Verification items for the finished model (mm, model axes). Face numbers are marked on the shaded views. A direction names the side the tool comes from. Coordinates: 2 decimals unless noted, no trailing zeros. Loops run counter-clockwise (first coordinate to the right, second up) from the corner with the lowest first, then second, coordinate; pieces in that order, holes last.
Q1. Access from +Z, -Z, +X, -X, +Y, -Y to the whole of each face (thin tool, end or side, straight path). Record for the marked faces 4 and 5.
Q2. Mould release check, pull along Z, two halves, no side actions. Record for the marked faces 1, 2 and 3: +Z half, -Z half, draft (parallel to the pull), parting line (faces both ways), or undercut.
Q3. Material ranges on probe 1 along Z at (x, y) = (-12.5, -12.25); probe 2 along X at (y, z) = (-2.5, -1); probe 3 along Z at (x, y) = (1.5, -8), recorded low to high.
Q4. Sectioned sample at A-A (x = 1). Enter the section's corners in (y, z).
Q5. Sectioned sample at B-B (z = 51). Enter the section's corners in (x, y), then the cut area to 3 significant figures.
Q6. Sectioned sample at D-D (y = -7). Count the separate pieces of the cut face and the enclosed holes in it, then the cut area to 3 significant figures.
Q7. Sectioned sample at C-C (z = 16). Enter the section's corners in (x, y).
Q8. Go/stop test with flat-tipped pins: P1, Ø0.9, axis at x = -12, z = 24.5, coming from the +Y side; P2, Ø0.5, axis at y = -7, z = 36.5, coming from the +X side; P3, Ø0.5, axis at x = -28.5, z = 46, coming from the +Y side. Record where each tip stops, or that it passes through.
```python
from build123d import *

# Parameters (mm, degrees)
BOSS_EXTRUDE1_DEPTH            = 77
SKETCH3_W                      = 37.54
SKETCH3_H                      = 17.27
BOSS_EXTRUDE2_DEPTH            = 1.77
SKETCH4_W                      = 37.54
SKETCH4_H                      = 17.27
BOSS_EXTRUDE3_DEPTH            = 1.77
SKETCH5_W                      = 4
SKETCH5_H                      = 16
CUT_EXTRUDE2_DEPTH             = 1.77
SKETCH6_W                      = 9.78
SKETCH6_H                      = 11.05
SKETCH6_W_2                    = 7.24
SKETCH6_H_2                    = 7.24
BUTTON_WALLS_DEPTH             = 7.24
SKETCH7_W                      = 9.78
SKETCH7_H                      = 11.05
BUTTON_BOTTOM_DEPTH            = 1.27
SKETCH8_W                      = 7.24
SKETCH8_H                      = 1.77
BUTTON_CUTOUT_MIDDLE_DEPTH     = 7.24
SKETCH9_W                      = 4.45
SKETCH9_H                      = 1.27
SKETCH9_W_2                    = 3.37
SKETCH9_H_2                    = 4.39
BUTTON_CUTOUT_FRONT_BACK_DEPTH = 7.24
SKETCH10_W                     = 3.37
SKETCH10_H                     = 4.39
BUTTON_CUTOUT_BOTTOM_DEPTH     = 1.27
BUTTON_CHAMFER1_SIZE           = 5
SKETCH12_W                     = 35
SKETCH12_H                     = 1.77
SKETCH12_W_2                   = 1.77
SKETCH12_H_2                   = 10
SKETCH12_W_3                   = 7.5
SKETCH12_R                     = 0.9652
SKETCH12_H_3                   = 7
SUPPORT_PCB_BATTERY_DEPTH      = 7
SKETCH13_R                     = 1.25
SKETCH13_W                     = 12
SKETCH13_H                     = 9
CUTOUT_USB_3_LEDS_DEPTH        = 1.77
SKETCH16_W                     = 1.77
SKETCH16_H                     = 1.77
TAB_PCB_RETAINER_LEN_DEPTH     = 3
SKETCH17_W                     = 4
SKETCH17_H                     = 1.77
CUTOUT_BACK_MOT_WIRES_DEPTH    = 9
SKETCH18_R                     = 1.25
CUTOUT_CHG_DONE_LED_DEPTH      = 10
SKETCH19_W                     = 4.2
SKETCH19_H                     = 1.77
TAB_PCB_RETAINERS_WIDTH_DEPTH  = 10
CUTOUT_RETAINER_TAB_1_DEPTH    = 1.77
CUTOUT_RETAINER_TAB_2_DEPTH    = 1.77


with BuildPart() as part:
    # Sketch2 → Boss-Extrude1 (new body)
    with BuildSketch(Plane.XY):
        Polygon((-30.215355805, 3.088014981), (-30.215355805, -12.911985019), (4.784644195, -12.911985019), (4.784644195, 3.088014981), (6.054644195, 3.088014981), (6.054644195, -14.181985019), (-31.485355805, -14.181985019), (-31.485355805, 3.088014981), align=None)
    extrude(amount=BOSS_EXTRUDE1_DEPTH)

    # Sketch3 → Boss-Extrude2 (add)
    with BuildSketch(Plane.XY.offset(77)):
        with Locations((-12.715355805, -5.546985019)):
            Rectangle(SKETCH3_W, SKETCH3_H)
    extrude(amount=BOSS_EXTRUDE2_DEPTH)

    # Sketch4 → Boss-Extrude3 (add)
    with BuildSketch(Plane(origin=(0, 0, 0), x_dir=(-1, 0, 0), z_dir=(0, 0, -1))):
        with Locations((12.715355805, -5.546985019)):
            Rectangle(SKETCH4_W, SKETCH4_H)
    extrude(amount=BOSS_EXTRUDE3_DEPTH)

    # Sketch5 → Cut-Extrude2 (cut)
    with BuildSketch(Plane(origin=(0, 0, -1.77), x_dir=(-1, 0, 0), z_dir=(0, 0, -1))):
        with Locations((19.215355805, -4.911985019)):
            Rectangle(SKETCH5_W, SKETCH5_H)
    extrude(amount=-CUT_EXTRUDE2_DEPTH, mode=Mode.SUBTRACT)

    # Sketch6 → button_walls (add)
    with BuildSketch(Plane(origin=(0, 3.088014981, 0), x_dir=(1, 0, 0), z_dir=(0, 1, 0))):
        with Locations((-7.725355805, 1.135)):
            Rectangle(SKETCH6_W, SKETCH6_H)
        with Locations((-7.725355805, 1.77)):
            Rectangle(SKETCH6_W_2, SKETCH6_H_2, mode=Mode.SUBTRACT)
    extrude(amount=-BUTTON_WALLS_DEPTH)

    # Sketch7 → button_bottom (add)
    with BuildSketch(Plane.XZ.offset(4.151985019)):
        with Locations((-7.725355805, -1.135)):
            Rectangle(SKETCH7_W, SKETCH7_H)
    extrude(amount=BUTTON_BOTTOM_DEPTH)

    # Sketch8 → button_cutout_middle (cut)
    with BuildSketch(Plane(origin=(0, 3.088014981, 0), x_dir=(1, 0, 0), z_dir=(0, 1, 0))):
        with Locations((-7.725355805, 0.885)):
            Rectangle(SKETCH8_W, SKETCH8_H)
    extrude(amount=-BUTTON_CUTOUT_MIDDLE_DEPTH, mode=Mode.SUBTRACT)

    # Sketch9 → button_cutout_front_back (cut)
    with BuildSketch(Plane(origin=(0, 3.088014981, 0), x_dir=(1, 0, 0), z_dir=(0, 1, 0))):
        with Locations((-7.720355805, 6.025)):
            Rectangle(SKETCH9_W, SKETCH9_H)
        with Locations((-10.930355805, -2.195)):
            Rectangle(SKETCH9_W_2, SKETCH9_H_2)
        with Locations((-4.520355805, -2.195)):
            Rectangle(SKETCH9_W_2, SKETCH9_H_2)
    extrude(amount=-BUTTON_CUTOUT_FRONT_BACK_DEPTH, mode=Mode.SUBTRACT)

    # Sketch10 → button_cutout_bottom (cut)
    with BuildSketch(Plane(origin=(0, -4.151985019, 0), x_dir=(1, 0, 0), z_dir=(0, 1, 0))):
        with Locations((-10.930355805, -2.195)):
            Rectangle(SKETCH10_W, SKETCH10_H)
        with Locations((-4.520355805, -2.195)):
            Rectangle(SKETCH10_W, SKETCH10_H)
    extrude(amount=-BUTTON_CUTOUT_BOTTOM_DEPTH, mode=Mode.SUBTRACT)

    # button_Chamfer1
    # the kernel refuses this chamfer: 5 mm, written as the material it adds along each edge
    with BuildSketch(Plane(origin=(-6.205355805, -5.421985019, 0), x_dir=(0, -0.9996219169112968, -0.027495876610586372), z_dir=(-1, 0, 0))) as button_chamfer1_piece_1_section:
        Polygon((BUTTON_CHAMFER1_SIZE * 0.999621916911, BUTTON_CHAMFER1_SIZE * 0.0274958766106), (-BUTTON_CHAMFER1_SIZE * 0.0274958766106, BUTTON_CHAMFER1_SIZE * 0.999621916911), (0, 0), align=None)
    button_chamfer1_piece_1 = extrude(amount=3.04, mode=Mode.PRIVATE)
    button_chamfer1_piece_1 = split(button_chamfer1_piece_1, bisect_by=Plane(origin=(-7.725355805, -7.110612501, 4.39), z_dir=(0, 0, -1)), keep=Keep.TOP, mode=Mode.PRIVATE)
    add(button_chamfer1_piece_1)

    # Sketch12 → support_pcb_battery (add)
    # profile 1 of 5: a face of its own
    with BuildSketch(Plane(origin=(0, -12.911985019, 0), x_dir=(1, 0, 0), z_dir=(0, 1, 0))):
        with Locations((-12.715355805, -76.115)):
            Rectangle(SKETCH12_W, SKETCH12_H)
    # profile 2 of 5: a face of its own
    with BuildSketch(Plane(origin=(0, -12.911985019, 0), x_dir=(1, 0, 0), z_dir=(0, 1, 0))):
        with Locations((-27.100355805, -60.23)):
            Rectangle(SKETCH12_W_2, SKETCH12_H_2)
    # profile 3 of 5: a face of its own
    with BuildSketch(Plane(origin=(0, -12.911985019, 0), x_dir=(1, 0, 0), z_dir=(0, 1, 0))):
        with Locations((1.034644195, -36.845)):
            Rectangle(SKETCH12_W_3, SKETCH12_H)
    # profile 4 of 5: a face of its own
    with BuildSketch(Plane(origin=(0, -12.911985019, 0), x_dir=(1, 0, 0), z_dir=(0, 1, 0))):
        with BuildLine():
            Line((-25.783918863, -37.73), (-19.764792747, -37.73))
            ThreePointArc((-19.764792747, -37.73), (-22.774355805, -30.7466), (-25.783918863, -37.73))
        make_face()
        with Locations(Location((-22.774355805, -34.8868, 0), (0, 0, 270))):
            Circle(SKETCH12_R, mode=Mode.SUBTRACT)
    # profile 5 of 5: a face of its own
    with BuildSketch(Plane(origin=(0, -12.911985019, 0), x_dir=(1, 0, 0), z_dir=(0, 1, 0))):
        with Locations((-12.100355805, -23.33)):
            Rectangle(SKETCH12_W_2, SKETCH12_H_3)
    extrude(amount=SUPPORT_PCB_BATTERY_DEPTH)

    # Sketch13 → cutout_usb_3_leds (cut)
    with BuildSketch(Plane(origin=(6.054644195, 0, 0), x_dir=(0, 0, -1), z_dir=(1, 0, 0))):
        with Locations((-51.3968, -3.411985019)):
            Circle(SKETCH13_R)
        with Locations((-47.5868, -3.411985019)):
            Circle(SKETCH13_R)
        with Locations((-24.2188, -3.411985019)):
            Circle(SKETCH13_R)
        with Locations((-34.8868, -3.411985019)):
            Rectangle(SKETCH13_W, SKETCH13_H)
    extrude(amount=-CUTOUT_USB_3_LEDS_DEPTH, mode=Mode.SUBTRACT)

    # Sketch16 → tab_pcb_retainer_len (add)
    with BuildSketch(Plane(origin=(0, -5.911985019, 0), x_dir=(1, 0, 0), z_dir=(0, 1, 0))):
        with Locations((-12.100355805, -20.715)):
            Rectangle(SKETCH16_W, SKETCH16_H)
    extrude(amount=TAB_PCB_RETAINER_LEN_DEPTH)

    # Sketch17 → cutout_back_mot_wires (cut)
    with BuildSketch(Plane(origin=(0, 3.088014981, 0), x_dir=(1, 0, 0), z_dir=(0, 1, 0))):
        with Locations((-20.361355805, -77.885)):
            Rectangle(SKETCH17_W, SKETCH17_H)
    extrude(amount=-CUTOUT_BACK_MOT_WIRES_DEPTH, mode=Mode.SUBTRACT)

    # Sketch18 → cutout_chg_done_led (cut)
    with BuildSketch(Plane(origin=(6.054644195, 0, 0), x_dir=(0, 0, -1), z_dir=(1, 0, 0))):
        with Locations((-28.5368, -3.411985019)):
            Circle(SKETCH18_R)
    extrude(amount=-CUTOUT_CHG_DONE_LED_DEPTH, mode=Mode.SUBTRACT)

    # Sketch19 → tab_pcb_retainers_width (add)
    with BuildSketch(Plane(origin=(0, -12.911985019, 0), x_dir=(1, 0, 0), z_dir=(0, 1, 0))):
        with Locations((-28.115355805, -68.615)):
            Rectangle(SKETCH19_W, SKETCH19_H)
        with Locations((-28.115355805, -46.115)):
            Rectangle(SKETCH19_W, SKETCH19_H)
        with Locations((-28.115355805, -28.115)):
            Rectangle(SKETCH19_W, SKETCH19_H)
    extrude(amount=TAB_PCB_RETAINERS_WIDTH_DEPTH)

    # Sketch20 → cutout_retainer_tab_1 (cut)
    with BuildSketch(Plane.XY.offset(69.5)):
        Polygon((-26.015355805, -12.911985019), (-26.015355805, -5.911985019), (-28.445355805, -10.120868481), (-28.445355805, -12.911985019), align=None)
    extrude(amount=-CUTOUT_RETAINER_TAB_1_DEPTH, mode=Mode.SUBTRACT)

    # Sketch21 → cutout_retainer_tab_2 (cut)
    with BuildSketch(Plane.XY.offset(47)):
        Polygon((-26.015355805, -5.911985019), (-28.445355805, -10.120868481), (-28.445355805, -12.911985019), (-26.015355805, -12.911985019), align=None)
    extrude(amount=-CUTOUT_RETAINER_TAB_2_DEPTH, mode=Mode.SUBTRACT)


solid = part.part
```
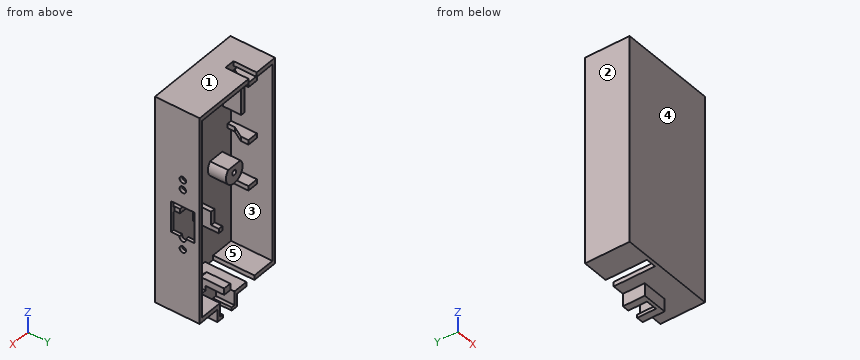
Geometry check:
1. face 4: +Z, -Z, +X, -X, -Y
1. face 5: +Y
2. face 1: +Z half
2. face 2: draft
2. face 3: undercut
3. probe 1: z = -1.77 to 0, 19.83 to 26.83, 75.23 to 78.77
3. probe 2: x = -31.49 to -21.22, -17.22 to -11.35, -4.11 to 6.05
3. probe 3: z = -1.77 to 0, 35.96 to 37.73, 75.23 to 78.77
4. outline: (-14.18, -1.77) - (3.09, -1.77) - (3.09, 0) - (-12.91, 0) - (-12.91, 35.96) - (-5.91, 35.96) - (-5.91, 37.73) - (-12.91, 37.73) - (-12.91, 75.23) - (-5.91, 75.23) - (-5.91, 77) - (3.09, 77) - (3.09, 78.77) - (-14.18, 78.77) - close
5. outline: (-31.49, -14.18) - (6.05, -14.18) - (6.05, -4.6) - (4.78, -4.6) - (4.78, -12.91) - (-30.22, -12.91) - (-30.22, 3.09) - (-31.49, 3.09) - close; (4.78, -2.23) - (6.05, -2.23) - (6.05, 3.09) - (4.78, 3.09) - close
5. area: 85.3 mm2
6. separate pieces: 6
6. enclosed holes: 1
6. area: 487 mm2
7. outline: (-31.49, -14.18) - (6.05, -14.18) - (6.05, 3.09) - (4.78, 3.09) - (4.78, -12.91) - (-30.22, -12.91) - (-30.22, 3.09) - (-31.49, 3.09) - close
8. P1: stops at y = -5.91
8. P2: stops at x = 4.28
8. P3: stops at y = -2.91
